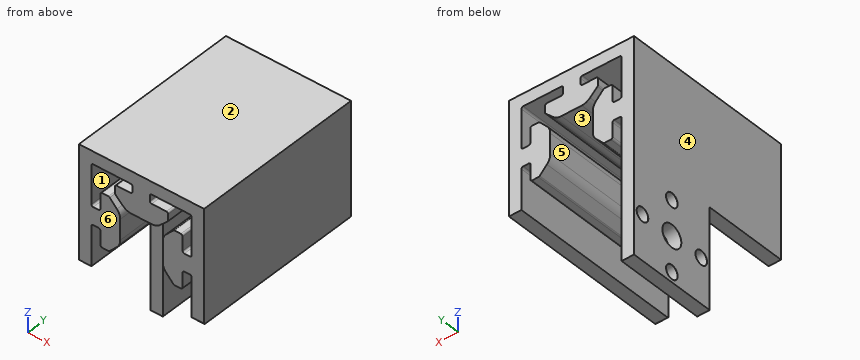
from build123d import *

# Parameters (mm, degrees)
BOSS_EXTRUDE1_DEPTH            = 70
FILLET4_R                      = 0.7
FILLET6_R                      = 4.8
FILLET12_R                     = 0.5
SKETCH2_W                      = 40
SKETCH2_H                      = 36
BOSS_EXTRUDE2_DEPTH            = 5
M5_CLEARANCE_HOLE1_D           = 5.5
M5_CLEARANCE_HOLE1_DEPTH       = 13
M5_CLEARANCE_HOLE1_CSINK_D     = 5.55
M5_CLEARANCE_HOLE1_CSINK_ANGLE = 90
M5_CLEARANCE_HOLE1_TIP         = 1.652366702
SKETCH7_R                      = 4.5
CUT_EXTRUDE1_DEPTH             = 46
CUT_EXTRUDE1_DEPTH_BACK        = 6


with BuildPart() as part:
    # Sketch1 → Boss-Extrude1 (new body)
    with BuildSketch(Plane(origin=(0, 0, 0), x_dir=(1, 0, 0), z_dir=(0, 1, 0))):
        Polygon((-25, -25), (25, -25), (25, 20), (20, 20), (20, 3.375), (16.42, 3.375), (16.42, 10.625), (12.92, 10.625), (8.5, 6), (8.5, -6), (12.92, -10.625), (16.42, -10.625), (16.42, -3.625), (20, -3.625), (20, -20), (3.375, -20), (3.375, -16.42), (10.625, -16.42), (10.625, -12.92), (6, -8.5), (-6, -8.5), (-10.625, -12.92), (-10.625, -16.42), (-3.625, -16.42), (-3.625, -20), (-20, -20), (-20, -3.375), (-16.42, -3.375), (-16.42, -10.625), (-12.92, -10.625), (-8.5, -6), (-8.5, 6), (-12.92, 10.625), (-16.42, 10.625), (-16.42, 3.625), (-20, 3.625), (-20, 20), (-25, 20), align=None)
    extrude(amount=BOSS_EXTRUDE1_DEPTH)

    # Fillet4
    fillet4_edges = [part.edges().sort_by_distance(p)[0] for p in [
        (-3.625, 35, 16.42),
        (-10.625, 35, 16.42),
        (-10.625, 35, 12.92),
        (10.625, 35, 12.92),
        (10.625, 35, 16.42),
        (3.375, 35, 16.42),
        (3.375, 35, 20),
        (20, 35, 20),
        (20, 35, 3.625),
        (16.42, 35, 3.625),
        (16.42, 35, 10.625),
        (12.92, 35, 10.625),
        (12.92, 35, -10.625),
        (16.42, 35, -10.625),
        (16.42, 35, -3.375),
        (20, 35, -3.375),
        (-20, 35, -3.625),
        (-16.42, 35, -3.625),
        (-16.42, 35, -10.625),
        (-12.92, 35, -10.625),
        (-12.92, 35, 10.625),
        (-16.42, 35, 10.625),
        (-16.42, 35, 3.375),
        (-20, 35, 3.375),
        (-20, 35, 20),
        (-3.625, 35, 20),
    ]]
    fillet(fillet4_edges, radius=FILLET4_R)

    # Fillet6
    fillet6_edges = [part.edges().sort_by_distance(p)[0] for p in [
        (-6, 35, 8.5),
        (6, 35, 8.5),
        (8.5, 35, 6),
        (8.5, 35, -6),
        (-8.5, 35, -6),
        (-8.5, 35, 6),
    ]]
    fillet(fillet6_edges, radius=FILLET6_R)

    # Fillet12
    fillet12_edges = [part.edges().sort_by_distance(p)[0] for p in [
        (22.5, 0, -20),
    ]]
    fillet(fillet12_edges, radius=FILLET12_R)

    # Sketch2 → Boss-Extrude2 (add)
    with BuildSketch(Plane.ZY.offset(25)):
        with Locations((-40, 52)):
            Rectangle(SKETCH2_W, SKETCH2_H)
    extrude(amount=-BOSS_EXTRUDE2_DEPTH)

    # M5 Clearance Hole1
    with Locations(Plane.ZY.offset(25)):
        with Locations((-56, 52), (-42, 66), (-28, 52), (-42, 38)):
            CounterSinkHole(M5_CLEARANCE_HOLE1_D / 2, M5_CLEARANCE_HOLE1_CSINK_D / 2, depth=M5_CLEARANCE_HOLE1_DEPTH, counter_sink_angle=M5_CLEARANCE_HOLE1_CSINK_ANGLE)
            with Locations((0, 0, -(M5_CLEARANCE_HOLE1_DEPTH + M5_CLEARANCE_HOLE1_TIP / 2))):  # 118° drill point
                Cone(0, M5_CLEARANCE_HOLE1_D / 2, M5_CLEARANCE_HOLE1_TIP, mode=Mode.SUBTRACT)

    # Sketch7 → Cut-Extrude1 (cut, two sides)
    with BuildSketch(Plane(origin=(-20, 0, 0), x_dir=(0, 0, -1), z_dir=(1, 0, 0))) as cut_extrude1_sk:
        with Locations((42, 52)):
            Circle(SKETCH7_R)
    extrude(amount=CUT_EXTRUDE1_DEPTH, mode=Mode.SUBTRACT)
    extrude(cut_extrude1_sk.sketch, amount=-CUT_EXTRUDE1_DEPTH_BACK, mode=Mode.SUBTRACT)


solid = part.part
Can you work these out from the model? Positions are in its coordinate system, mm. Face numbers are marked on the shaded views. A direction names the side the tool comes from. Round coordinates to 2 decimals unless told otherwise and drop trailing zeros. Write each loop counter-clockwise with the first axis right and the second up, starting at its lowest first coordinate (ties: lowest second). Pieces come first, ordered by that corner, then holes. Notation, with made-up numbers: M 55.5,67.25 L 114.5,67.25 A20 ccw 114.5,94.25 Z; hole C 76,-22 d1. An arc over 180 degrees is marked long. Use CSV: the item, a comma, the result in double quotes.
(1) I'm going to push flat-ended pins straight in: pin 1 (5.5 mm diameter, centred on x = -22.5, z = -40.5, fed in from -Y); pin 2 (1.3 mm diameter, centred on x = -14, y = 37.5, fed in from -Z) (3 decimals); pin 3 (3 mm diameter, centred on x = 8, y = 12, fed in from -Z); pin 4 (7 mm diameter, centred on y = 52, z = -42, fed in from +X). Where does each tip first touch, or does it pass through?
Check values:
pin 1,"y = 34"
pin 2,"z = -10.625"
pin 3,"z = -7.01"
pin 4,"through"
(2) Imagine slicing it at C-C (y = 52). Count the separate pieces of the cut face and the enclosed holes in it, plus the area to 3 significant figures.
Check values:
separate pieces,"4"
enclosed holes,"0"
area,"1,270 mm^2"
(3) We'd pull the mould along X, two halves only. Please class the marked faces 4, 5 and 6: +X half, -X half, draft (parallel to the pull), parting line (faces both ways), or undercut.
Check values:
face 4,"-X half"
face 5,"undercut"
face 6,"draft"
(4) On a 3-axis mill with a long thin cutter (end or side, diameter ignored), from which of +Z, -Z, +X, -X, +Y, -Y can I reach the whole of each face in a straight line? I mean the marked faces 1, 2 and 3. Say none if no direction works.
Check values:
face 1,"+Y, -Y"
face 2,"+Z, +X, -X, +Y, -Y"
face 3,"-Z, +Y, -Y"
(5) Imagine slicing it at B-B (z = -42). Write out the boundary of the cut face in (x, y) (3 decimals).
Check values:
outline,"M -25,34 L -20,34 L -20,35.25 L -24.975,35.25 L -25,35.225 Z; M -25,40.775 L -24.975,40.75 L -20,40.75 L -20,47.5 L -25,47.5 Z; M -25,56.5 L -20,56.5 L -20,63.25 L -24.975,63.25 L -25,63.225 Z; M -25,68.775 L -24.975,68.75 L -20,68.75 L -20,70 L -25,70 Z"
(6) Imagine slicing it at D-D (z = -17). Write out the boundary of the cut face in (x, y), plus the area to 3 significant figures.
Check values:
outline,"M -25,0 L -20,0 L -20,70 L -25,70 Z; M 20,0 L 25,0 L 25,70 L 20,70 Z"
area,"700 mm^2"
(7) I need wall thicknesses on line 1 along Y through (x, z) = (-21, -42); line 2 along Z through (x, y) = (-22, 66); line 3 along X through (y, z) = (63, -0.5). Which ranges of each line are inside material? Lowest first, please.
Check values:
line 1,"34 to 35.25, 40.75 to 47.5, 56.5 to 63.25, 68.75 to 70"
line 2,"-60 to -44.75, -39.25 to 25"
line 3,"-25 to -8.5, 8.5 to 25"
(8) Imagine slicing it at A-A (z = -28). Write out the boundary of the cut face in (x, y) (3 decimals), plus the area to 3 significant figures.
Check values:
outline,"M -25,34 L -20,34 L -20,49.25 L -24.975,49.25 L -25,49.225 Z; M -25,54.775 L -24.975,54.75 L -20,54.75 L -20,70 L -25,70 Z"
area,"152 mm^2"
